Autodesk Inventor part; units mm, degrees
ref_plane "Cross Section Plane" through (33.176, 21.6358, 0) normal (-0.5013, 0.8653, 0) x (0, 0, 1)
ref_plane "YZ Plane" through (0, 0, 0) normal (1, 0, 0) x (0, 1, 0)
ref_plane "XZ Plane" through (0, 0, 0) normal (0, 1, 0) x (-1, 0, 0)
sketch "Sketch Path" plane through (0, 0, 0) normal (0, 0, 1) x (1, 0, 0)
  arc A0 (-4.9901, -38.2586) -> (33.176, 21.6358) centre (-1.4345, 1.5831) ccw
  arc A1 (-169.8676, 372.0838) -> (-408.4059, -2.2563) centre (-386.1833, 246.7541) ccw
  line L0 (-169.8676, 372.0838) -> (33.176, 21.6358)
  line L1 (-4.9901, -38.2586) -> (-408.4059, -2.2563)
ref_plane "Cross Section Plane" through (33.176, 21.6358, 0) normal (-0.5013, 0.8653, 0) x (0, 0, 1)
sketch "Cross Section" plane through (33.176, 21.6358, 0) normal (-0.5013, 0.8653, 0) x (0, 0, 1)
  line L0 (0, 2.4986) -> (0, -3.5014) construction
  line L1 (-4.25, 0) -> (4.25, 0) construction
  line L2 (-5.1594, 2.4986) -> (5.1594, 2.4986)
  line L3 (5.1594, 2.4986) -> (2.9756, -3.5014)
  line L4 (2.9756, -3.5014) -> (-2.9756, -3.5014)
  line L5 (-2.9756, -3.5014) -> (-5.1594, 2.4986)
  point P0 (0, 0)
  point P1 (0, 0)
  point P2 (0, 0)
  dimension "d0" = 8.5
  dimension "d1" = 2.4986
  dimension "d2" = 40
  dimension "d3" = 6
sweep "Belt" add profiles "Cross Section" path "Sketch Path"
equation "\"d0\" = da_Bw"
equation "\"d1\" = da_Hw"
equation "\"d2\" = da_Alfa"
equation "\"d3\" = da_H"
equation "\"da_Alfa\" = 40deg"
equation "\"da_H\" = 6"
equation "\"da_Bw\" = 8.5"
equation "\"da_Hw\" = 2.49859"
properties part number "V-Belt" material "Rubber"
Check sheet for the modelled part. Datum: model origin and axes. Units: mm. A direction names the side the tool comes from. Coordinates: 2 decimals unless noted, no trailing zeros. Write each loop counter-clockwise with the first axis right and the second up, starting at its lowest first coordinate (ties: lowest second). Pieces come first, ordered by that corner, then holes. Notation, with made-up numbers: (24.25, 82) - (31.25, 82) arc R18 cw to (31.25, 97) - close; hole circle Ø11 at (47.25, 0). An arc over 180 degrees is marked (long way). One line per question, with ' | ' between items.
Item 1: Gauge pin test, flat ends, axial feed: P1, Ø3, axis at y = 303, z = -2, coming from the +X side; P2, Ø5, axis at x = -371, z = 1, coming from the +Y side; P3, Ø4, axis at y = 84, z = -1.5, coming from the -X side. Record the tip position at first contact, or that the pin passes through.
Determined:
P1: stops at x = -126.08 | P2: stops at y = 498.93 | P3: stops at x = -580.9
Item 2: Sectioned sample at A-A on x = -29.5. Record the boundary of the cut face in (y, z).
Determined:
outline: (-38.58, -5.16) - (-32.56, -2.98) - (-32.56, 2.98) - (-38.58, 5.16) - close; (122.83, -2.98) - (134.8, -5.16) - (134.8, 5.16) - (122.83, 2.98) - close
Item 3: Sectioned sample at B-B on z = 1.25. Record the boundary of the cut face in (x, y) (3 decimals).
Determined:
outline: (-408.628, -4.745) - (-5.212, -40.747) arc R42.499 ccw to (35.338, 22.888) - (-167.706, 373.336) arc R252.499 ccw (long way) to start; hole (-408.095, 1.231) - (-4.679, -34.771) arc R36.499 ccw to (30.146, 19.881) - (-172.897, 370.329) arc R246.499 ccw (long way) to start
Item 4: Access from +Z, -Z, +X, -X, +Y, -Y to the whole of each face (thin tool, end or side, straight path). Record for faces 4 (the face through (-70.164, 199.083, -4.083)), 5 (the face through (-70.24, 199.04, 4.05)), 6 (the face through (29.04, -18.5, 0.04)).
Determined:
face 4: -Z | face 5: +Z | face 6: +Z, -Z
Item 5: Mould release check, pull along Y, two halves, no side actions. Record for faces 1 (the face through (-602.93, 376.28, -0.07)), 2 (the face through (-590.2, 385.1, 0)), 3 (the face through (-204.096, -22.998, 0.072)): pulls with the +Y half, pulls with the -Y half, needs draft (parallel to the pull), parting line crosses it, or undercut.
Determined:
face 1: parting line crosses it | face 2: undercut | face 3: pulls with the -Y half
Item 6: Thickness scan on line 1 (X direction, y = 259.5, z = 1.25); line 2 (Y direction, x = -91, z = 1); line 3 (Y direction, x = -208, z = 2.5). Record the ranges inside material, lowest first. Write a range as [from, to].
Determined:
line 1: x = [-638.36, -632.35], [-108.69, -101.75] | line 2: y = [-33.09, -27.07], [228.98, 240.94] | line 3: y = [-22.65, -16.63], [417.08, 425.66]
